Can you work these out from the model? Positions are in its coordinate system, mm. Face numbers are marked on the shaded views. Round coordinates to 2 decimals unless told otherwise and drop trailing zeros. Order: outer loops, then holes, each group sorted by start corner. A loop starts at its lowest first (then second) coordinate and runs counter-clockwise, first axis right, second up. Notation, with made-up numbers: M -9.5,80.25 L 7.5,80.25 A19 ccw 7.5,90.25 Z; hole C 34,57.25 d7. An arc over 180 degrees is marked long. Answer as a JSON object with one key per item and string values. Group by question number.
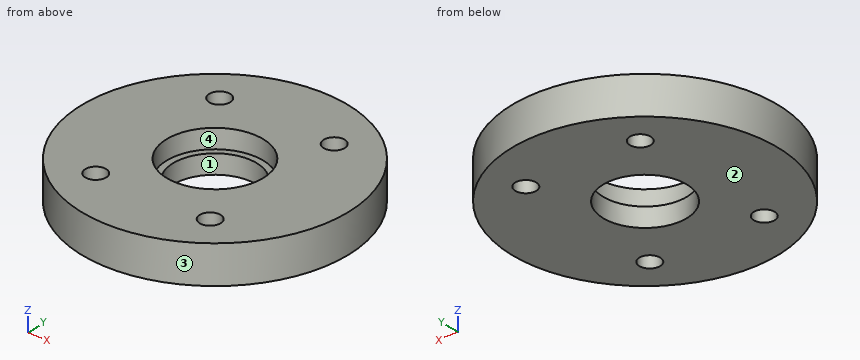
```python
from build123d import *

# Parameters (mm, degrees)
F2_R     = 2.75
F3_DEPTH = 10


with BuildPart() as f1:
    # F0 (on Front) → F1 (revolve)
    with BuildSketch(Plane.XZ):
        Polygon((11, 5), (11, 0), (35, 0), (35, 10), (12.7, 10), (12.7, 5), align=None)
    revolve(axis=Axis((0, 0, 6.447879), (0, 0, 1)))

    # F2 (on face) → F3 (cut)
    with BuildSketch(Plane.XY.offset(10)):
        with Locations((-15, 20)):
            Circle(F2_R)
        with Locations((-15, -20)):
            Circle(F2_R)
        with Locations((15, -20)):
            Circle(F2_R)
        with Locations((15, 20)):
            Circle(F2_R)
    extrude(amount=-F3_DEPTH, mode=Mode.SUBTRACT)


solid = f1.part
```
1) I need wall thicknesses on line 1 along X through (y, z) = (-21, 2.5); line 2 along Y through (x, z) = (-15, 3.25); line 3 along Y through (x, z) = (0, 8.85). Which ranges of each line are inside material? Lowest first, please.
2) We'd pull the mould along X, two halves only. Please class the marked faces 1, 2, 3 and 4: +X half, -X half, draft (parallel to the pull), parting line (faces both ways), or undercut.
3) If we section it at C-C on y = -20: Write out the boundary of the cut face in (x, z), plus the area to 3 significant figures.
4) If we section it at A-A on y = 0: Write out the boundary of the cut face in (x, z), plus the area to 3 significant figures.
5) For pin 1 (7 mm diameter, centred on x = 15, y = -20, fed in from -Z); pin 2 (4.5 mm diameter, centred on x = -15, y = 20, fed in from +Z); pin 3 (5 mm diameter, centred on x = 25.5, z = 3, fed in from +Y); pin 4 (4 mm diameter, centred on y = -9, z = 5.5, fed in from +X), each with a flat end and sliding along its axis, tell me the tip position at first contact or that it passes through.
6) If we section it at D-D on x = -15: Write out the boundary of the cut face in (y, z).
7) If we section it at B-B on z = 7.5: Write out the boundary of the cut face in (x, y), plus the area to 3 significant figures.
Findings:
{
 "1": {"line 1": "x = -28 to -17.56, -12.44 to 12.44, 17.56 to 28", "line 2": "y = -31.62 to -22.75, -17.25 to 17.25, 22.75 to 31.62", "line 3": "y = -35 to -12.7, 12.7 to 35"},
 "2": {"face 1": "undercut", "face 2": "draft", "face 3": "parting line", "face 4": "undercut"},
 "3": {"outline": "M -28.72,0 L -17.75,0 L -17.75,10 L -28.72,10 Z; M -12.25,0 L 12.25,0 L 12.25,10 L -12.25,10 Z; M 17.75,0 L 28.72,0 L 28.72,10 L 17.75,10 Z", "area": "464 mm^2"},
 "4": {"outline": "M -35,0 L -11,0 L -11,5 L -12.7,5 L -12.7,10 L -35,10 Z; M 11,0 L 35,0 L 35,10 L 12.7,10 L 12.7,5 L 11,5 Z", "area": "463 mm^2"},
 "5": {"pin 1": "stops at z = 0", "pin 2": "passes through", "pin 3": "stops at y = 26.38", "pin 4": "stops at x = 34.29"},
 "6": {"outline": "M -31.62,0 L -22.75,0 L -22.75,10 L -31.62,10 Z; M -17.25,0 L 17.25,0 L 17.25,10 L -17.25,10 Z; M 22.75,0 L 31.62,0 L 31.62,10 L 22.75,10 Z"},
 "7": {"outline": "C 0,0 d70; hole C -15,-20 d5.5; hole C -15,20 d5.5; hole C 0,0 d25.4; hole C 15,-20 d5.5; hole C 15,20 d5.5", "area": "3,250 mm^2"}
}
